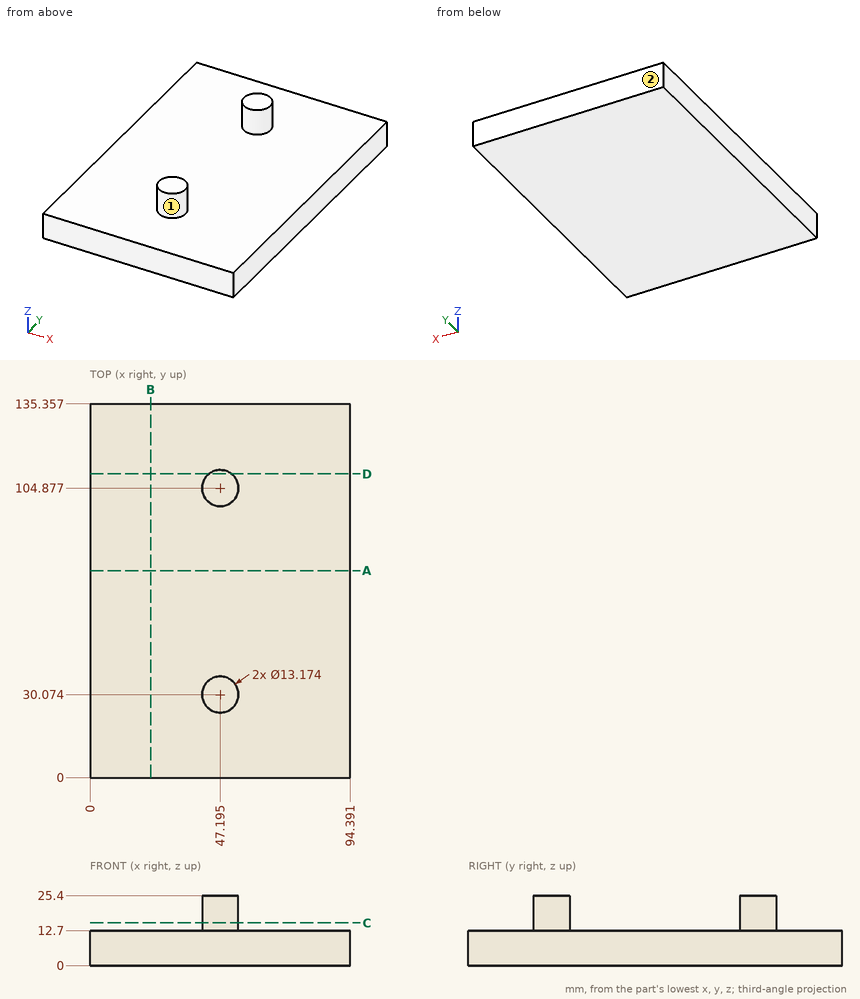
Verification items for this drawing (mm, ordinates from the low corner). A direction names the side the tool comes from. Give positions to 0.01 mm unless a question says otherwise; leave off trailing zeros. Write each loop counter-clockwise with the first axis right and the second up, starting at its lowest first coordinate (ties: lowest second). Pieces come first, ordered by that corner, then holes. Notation, with made-up numbers: (58, 33) -> (96, 33) arc R9 cw to (96, 42) -> close; hole circle Ø4 at (-23, -1). An arc over 180 degrees is marked (long way). Use CSV: the item, a comma, the result in double quotes.
(1) Material ranges on L1, parallel to Z at x = 17, y = 12; L2, parallel to X at y = 31, z = 23.5 (1 decimal), recorded low to high.
Derived:
L1,"z = 0 to 12.7"
L2,"x = 40.7 to 53.7"
(2) Sectioned sample at A-A (y = 75). Record the cut outline in (x, z).
Derived:
outline,"(0, 0) -> (94.39, 0) -> (94.39, 12.7) -> (0, 12.7) -> close"
(3) Go/stop test with flat-tipped pins: pin 1 (2 mm diameter, centred on x = 37, y = 75, fed in from -Z); pin 2 (2 mm diameter, centred on x = 13, y = 83, fed in from +Z). Record where each tip stops, or that it passes through.
Derived:
pin 1,"stops at z = 0"
pin 2,"stops at z = 12.7"
(4) Sectioned sample at C-C (z = 15.5). Record the cut outline in (x, y) (1 decimal), plus the area to 3 significant figures.
Derived:
outline,"circle Ø13.2 at (47.2, 30.1); circle Ø13.2 at (47.2, 104.9)"
area,"273 mm^2"
(5) Sectioned sample at D-D (y = 110). Record the cut outline in (x, z) (1 decimal), plus the area to 3 significant figures.
Derived:
outline,"(0, 0) -> (94.4, 0) -> (94.4, 12.7) -> (51.3, 12.7) -> (51.3, 25.4) -> (43.1, 25.4) -> (43.1, 12.7) -> (0, 12.7) -> close"
area,"1,300 mm^2"
(6) Set-up check for the marked faces 1 and 2: record each of +Z, -Z, +X, -X, +Y, -Y from which the full face is reachable in a straight line by a thin tool's end or side.
Derived:
face 1,"+Z"
face 2,"+Z, -Z, +X, -X, +Y"
(7) Sectioned sample at B-B (x = 22). Record the cut outline in (y, z), plus the area to 3 significant figures.
Derived:
outline,"(0, 0) -> (135.36, 0) -> (135.36, 12.7) -> (0, 12.7) -> close"
area,"1,720 mm^2"
